Verification items for the finished model (mm, model axes). A direction names the side the tool comes from. Round coordinates to 2 decimals unless told otherwise and drop trailing zeros. Write each loop counter-clockwise with the first axis right and the second up, starting at its lowest first coordinate (ties: lowest second). Pieces come first, ordered by that corner, then holes. Notation, with made-up numbers: (59, -19.5) -> (91, -19.5) arc R14 cw to (91, -5.5) -> close; hole circle Ø11 at (-21.5, 2.25). An arc over 180 degrees is marked (long way). Use CSV: the item, a comma, the result in double quotes.
Autodesk Inventor part; units mm, degrees
ref_plane "Work Plane1" through (0, 0, 10) normal (0, 0, 1) x (1, 0, 0)
ref_plane "Work Plane3" through (3.9701, 45.8299, 26) normal (1, 0, 0) x (0, -1, 0)
ref_plane "Work Plane4" through (-34.8055, 8.3289, 16.6138) normal (0.7071068, -0.7071068, 0) x (0.7071068, 0.7071068, 0)
ref_plane "Work Plane1" through (0, 0, 10) normal (0, 0, 1) x (1, 0, 0)
sketch "Sketch1" plane through (0, 0, 10) normal (0, 0, 1) x (1, 0, 0)
  line L0 (-4.0299, -0.3538) -> (-2.2322, 1.4439) construction
  arc A0 (-1.4439, 2.2322) -> (-2.2322, 1.4439) centre (-0.9299, 0.9299) ccw construction
  line L1 (-1.4439, 2.2322) -> (0.3538, 4.0299) construction
  line L2 (-37.8299, 42.8299) -> (-37.8299, 37.8299) construction
  line L3 (-37.8299, 37.8299) -> (-42.9208, 37.8299) construction
  line L4 (-37.8299, 42.2137) -> (-37.8299, 45.8299) construction
  line L5 (-37.8299, 45.8299) -> (-4.0299, 45.8299) construction
  line L6 (-4.0299, 45.8299) -> (-4.0299, 42.2137) construction
  line L7 (-4.0299, 4.0299) -> (0.3538, 4.0299)
  circle A1 centre (-20.9299, 20.9299) radius 17.5
  line L8 (-20.9299, 58.9723) -> (17.1124, 20.9299) construction
  line L9 (17.1124, 20.9299) -> (-20.9299, -17.1124) construction
  line L10 (-20.9299, -17.1124) -> (-58.9723, 20.9299) construction
  line L11 (-58.9723, 20.9299) -> (-20.9299, 58.9723) construction
  line L12 (-20.9299, 58.9723) -> (-20.9299, -17.1124) construction
  line L13 (17.1124, 20.9299) -> (-58.9723, 20.9299) construction
  line L14 (-20.9299, 58.9723) -> (32.8701, 58.9723) construction
  line L15 (-43.4299, 43.4299) -> (1.5701, 43.4299) construction
  line L16 (1.5701, 43.4299) -> (1.5701, -1.5701) construction
  line L17 (1.5701, -1.5701) -> (-43.4299, -1.5701) construction
  line L18 (-43.4299, -1.5701) -> (-43.4299, 43.4299) construction
  line L19 (-43.4299, 43.4299) -> (1.5701, -1.5701) construction
  line L20 (1.5701, 43.4299) -> (-43.4299, -1.5701) construction
  line L21 (-43.4299, 5.3876) -> (-43.4299, 36.4723)
  line L22 (-43.4299, 36.4723) -> (-36.4723, 43.4299)
  line L23 (-36.4723, 43.4299) -> (-5.3876, 43.4299)
  line L24 (-5.3876, 43.4299) -> (1.5701, 36.4723)
  line L25 (1.5701, 36.4723) -> (1.5701, 5.3876)
  line L26 (1.5701, 5.3876) -> (-5.3876, -1.5701)
  line L27 (-5.3876, -1.5701) -> (-36.4723, -1.5701)
  line L28 (-36.4723, -1.5701) -> (-43.4299, 5.3876)
  line L29 (-4.0299, 42.2137) -> (-37.8299, 42.2137)
  line L30 (-4.0299, -0.3538) -> (-4.0299, 4.0299)
  circle A2 centre (-20.9299, 20.9299) radius 1.4
  line L31 (-10.9299, 10.9299) -> (-30.9299, 10.9299) construction
  line L32 (-30.9299, 10.9299) -> (-30.9299, 30.9299) construction
  line L33 (-30.9299, 30.9299) -> (-10.9299, 30.9299) construction
  line L34 (-10.9299, 30.9299) -> (-10.9299, 10.9299) construction
  line L35 (-10.9299, 10.9299) -> (-30.9299, 30.9299) construction
  line L36 (-30.9299, 10.9299) -> (-10.9299, 30.9299) construction
  circle A3 centre (-30.9299, 30.9299) radius 1.4
  circle A4 centre (-30.9299, 10.9299) radius 1.4
  circle A5 centre (-10.9299, 10.9299) radius 1.4
  line L37 (-45.8299, 37.8299) -> (-42.0723, 37.8299) construction
  line L38 (-42.1723, 37.7299) -> (-45.8299, 37.7299)
  line L39 (-45.8299, 37.7299) -> (-45.8299, 4.1299)
  line L40 (-45.8299, 4.1299) -> (-42.1723, 4.1299)
  line L41 (-42.1723, 4.1299) -> (-42.1723, 37.7299)
  line L42 (-45.8299, 4.0299) -> (-42.0723, 4.0299) construction
  line L43 (-45.8299, 37.8299) -> (-42.0723, 37.8299)
  line L44 (-37.7299, 45.8299) -> (-4.1299, 45.8299)
  line L45 (-4.1299, 45.8299) -> (-4.1299, 42.1723)
  line L46 (-4.1299, 42.1723) -> (-37.7299, 42.1723)
  line L47 (-37.7299, 42.1723) -> (-37.7299, 45.8299)
  line L48 (0.4701, 37.8299) -> (0.4701, 4.0299) construction
  line L49 (0.4701, 4.0299) -> (3.9701, 4.0299) construction
  line L50 (3.9701, 37.8299) -> (3.9701, 4.0299) construction
  line L51 (0.4701, 37.8299) -> (3.9701, 37.8299) construction
  line L52 (-45.8299, -3.9701) -> (-4.0299, -3.9701) construction
  line L53 (0.3124, 37.7299) -> (3.9701, 37.7299)
  line L54 (3.9701, 37.7299) -> (3.9701, 4.1299)
  line L55 (3.9701, 4.1299) -> (0.3124, 4.1299)
  line L56 (0.3124, 4.1299) -> (0.3124, 37.7299)
  line L57 (-4.1713, -0.3538) -> (-37.7299, -0.3538)
  line L58 (-37.7299, -0.3538) -> (-37.7299, -3.9701)
  line L59 (-37.7299, -3.9701) -> (-4.1713, -3.9701)
  line L60 (-4.1713, -3.9701) -> (-4.1713, -0.3538)
  point P0 (-37.8299, 4.0299)
  dimension "d18" = 53.8
  dimension "d19" = 45
  dimension "d20" = 53.8
  dimension "d21" = 45
  dimension "d22" = 45
  dimension "d30" = 20
  dimension "d31" = 20
  dimension "d32" = 2.8
  dimension "d33" = 2.8
  dimension "d34" = 2.8
  dimension "d35" = 2.8
  dimension "d36" = 0.1
  dimension "d37" = 0.1
  dimension "d38" = 0.1
  dimension "d39" = 0.1
extrude "Extrusion1" add sketch "Sketch1" along normal blind 5 contours L30 L26 L57 L28 L41 L22 L46 L24 L56 L7 | L7 L26 L30 | L56 L24 L25 L26 | L26 L25 L24 L53 L54 L55 | L60 L59 L58 L57 L28 L27 L26 | L26 L27 L28 L57 | L46 L22 L29 L24 | L24 L29 L45 | L40 L39 L38 L22 L21 L28 | L28 L21 L22 L41 | L29 L22 L23 L24 | L24 L23 L22 L29 L47 L44 L45 | L47 L29 L22 | A1 | A2 | A3 | A4 | A5
sketch "Sketch4" plane through (0, 0, 15) normal (0, 0, 1) x (1, 0, 0)
  line L0 (-37.7299, 42.1723) -> (-42.1723, 37.7299)
  line L1 (-42.1723, 37.7299) -> (-45.8299, 37.7299)
  line L2 (-45.8299, 37.7299) -> (-45.8299, 4.1299)
  line L3 (-45.8299, 4.1299) -> (-42.1723, 4.1299)
  line L4 (-42.1723, 4.1299) -> (-37.6885, -0.3538)
  line L5 (-37.6885, -0.3538) -> (-37.7299, -0.3538)
  line L6 (-37.7299, -0.3538) -> (-37.7299, -3.9701)
  line L7 (-37.7299, -3.9701) -> (-4.1713, -3.9701)
  line L8 (-4.1713, -3.9701) -> (-4.1713, -0.3538)
  line L9 (-4.1713, -0.3538) -> (0.3124, 4.1299)
  line L10 (0.3124, 4.1299) -> (3.9701, 4.1299)
  line L11 (3.9701, 4.1299) -> (3.9701, 37.7299)
  line L12 (3.9701, 37.7299) -> (0.3124, 37.7299)
  line L13 (0.3124, 37.7299) -> (-4.1299, 42.1723)
  line L14 (-4.1299, 42.1723) -> (-4.1299, 45.8299)
  line L15 (-4.1299, 45.8299) -> (-37.7299, 45.8299)
  line L16 (-37.7299, 45.8299) -> (-37.7299, 42.1723)
  line L17 (-45.8299, 37.7299) -> (-45.8299, 4.1299)
  line L18 (-45.8299, 7.911) -> (-7.911, 45.8299)
  line L19 (-45.8299, 7.911) -> (7.7955, 7.911) construction
  line L20 (-7.911, 45.8299) -> (-14.9821, 45.8299)
  line L21 (-4.1299, 45.8299) -> (-37.7299, 45.8299)
  line L22 (-14.9821, 45.8299) -> (-45.8299, 14.9821)
  line L23 (-45.8299, 7.911) -> (-45.8299, 14.9821)
  circle A0 centre (-40.9299, 0.9299) radius 1.1933
  line L24 (0.3124, 37.7299) -> (-4.1299, 42.1723)
  point P0 (0, 0)
  dimension "d40" = 45
  dimension "d41" = 5
extrude "Extrusion4" add sketch "Sketch4" along normal blind 27.5 contours L15 L18 L2 L22
sketch "Sketch5" plane through (-45.8299, 14.9821, 15) normal (-0.7071068, 0.7071068, 0) x (-0.7071068, -0.7071068, 0)
  line L0 (0, 0) -> (-43.6254, 0)
  line L1 (0, 0) -> (0, 27.5)
  line L2 (-43.6254, 27.5) -> (0, 27.5)
  line L3 (-43.6254, 0) -> (-43.6254, 27.5)
  circle A0 centre (-21.8127, 5.6873) radius 21.8127
  line L4 (-6.8127, 24) -> (-36.8127, 24) construction
  line L5 (-36.8127, 24) -> (-36.8127, 4) construction
  line L6 (-36.8127, 4) -> (-6.8127, 4) construction
  line L7 (-6.8127, 4) -> (-6.8127, 24) construction
  line L8 (-6.8127, 24) -> (-36.8127, 4) construction
  line L9 (-36.8127, 24) -> (-6.8127, 4) construction
  point P0 (-21.8127, -15)
  point P1 (-21.8127, 14)
  dimension "d44" = 30
  dimension "d45" = 20
hole "Hole1" at (-19.7994, 41.0126, 39) at (-19.7994, 41.0126, 19) at (-41.0126, 19.7994, 39) at (-30.406, 30.406, 29) direction (0.7071068, -0.7071068, 0) diameter 2.8 depth 12
sketch "Sketch6" plane through (-37.7299, -3.9701, 10) normal (0, -1, 0) x (1, 0, 0)
  circle A0 centre (-3.2, 36.9) radius 1.45
  circle A1 centre (36.8, 36.9) radius 1.45
  line L0 (-6.1, 0) -> (-6.1, 39.8)
  line L1 (-0.1, 0) -> (-6.1, 0)
  line L2 (-0.1, 33.8) -> (-0.1, 0)
  line L3 (33.7, 33.8) -> (-0.1, 33.8)
  line L4 (33.7, 33.8) -> (33.7, 0)
  line L5 (39.7, 0) -> (33.7, 0)
  line L6 (39.7, 39.8) -> (39.7, 0)
  line L7 (-6.1, 39.8) -> (39.7, 39.8)
  circle A2 centre (16.8, 16.9) radius 16.9
  circle A3 centre (16.8, 16.9) radius 14.9
  line L8 (-0.1, 16.9) -> (-0.1, 0)
  line L9 (0, 0) -> (33.5586, 0)
  line L10 (0.0414, 0) -> (-4.4423, 0)
  line L11 (33.5586, 0) -> (0.0414, 0)
  line L12 (33.7, 16.9) -> (33.5586, 0)
  point P0 (37.7299, -10)
  dimension "d53" = 2
extrude "Extrusion5" cut sketch "Sketch6" against normal up to surface contours A3 surface through (-45.8299, 7.911, 15) normal (0.7071068, -0.7071068, 0)
ref_plane "Work Plane3" through (3.9701, 45.8299, 26) normal (1, 0, 0) x (0, -1, 0)
sketch "Sketch7" plane through (3.9701, 45.8299, 26) normal (1, 0, 0) x (0, -1, 0)
  line L0 (41.8, -17.8) -> (41.8, 16)
  line L1 (8, -17.8) -> (41.8, -17.8)
  line L2 (8, -17.8) -> (8, 16)
  circle A0 centre (24.9, -0.9) radius 16.9
  circle A1 centre (24.9, -0.9) radius 14.9
  point P0 (45.8299, 26)
  dimension "d56" = 2
ref_plane "Work Plane4" through (-34.8055, 8.3289, 16.6138) normal (0.7071068, -0.7071068, 0) x (0.7071068, 0.7071068, 0)
extrude "Extrusion6" cut sketch "Sketch7" against normal up to surface contours A1 surface through (-45.8299, 7.911, 15) normal (0.7071068, -0.7071068, 0)
sketch "Skizze8" plane through (0, 0, 10) normal (0, 0, -1) x (-1, 0, 0)
  line L0 (42.1723, 37.7299) -> (37.7299, 42.1723)
  line L1 (37.7299, 45.8299) -> (37.7299, 42.1723)
  line L2 (4.1299, 45.8299) -> (37.7299, 45.8299) construction
  line L3 (4.1299, 42.1723) -> (4.1299, 45.8299)
  line L4 (4.1299, 42.1723) -> (-0.3124, 37.7299)
  line L5 (-3.9701, 37.7299) -> (-0.3124, 37.7299)
  line L6 (-3.9701, 4.1299) -> (-3.9701, 37.7299) construction
  line L7 (-0.3124, 4.1299) -> (-3.9701, 4.1299)
  line L8 (-0.3124, 4.1299) -> (4.1713, -0.3538)
  line L9 (4.1713, -3.9701) -> (4.1713, -0.3538)
  line L10 (37.7299, -3.9701) -> (4.1713, -3.9701) construction
  line L11 (37.7299, -0.3538) -> (37.7299, -3.9701)
  line L12 (37.6885, -0.3538) -> (37.7299, -0.3538)
  line L13 (37.6885, -0.3538) -> (42.1723, 4.1299)
  line L14 (45.8299, 4.1299) -> (42.1723, 4.1299)
  line L15 (45.8299, 37.7299) -> (45.8299, 4.1299) construction
  line L16 (42.1723, 37.7299) -> (45.8299, 37.7299)
  line L17 (46.0299, 3.9299) -> (42.2551, 3.9299)
  line L18 (42.2551, 3.9299) -> (37.9299, -0.3953)
  line L19 (37.9299, -0.3953) -> (37.9299, -4.1701)
  line L20 (37.9299, -4.1701) -> (3.9713, -4.1701) construction
  line L21 (3.9713, -4.1701) -> (3.9713, -0.4367)
  line L22 (3.9713, -0.4367) -> (-0.3953, 3.9299)
  line L23 (-0.3953, 3.9299) -> (-4.1701, 3.9299)
  line L24 (-4.1701, 3.9299) -> (-4.1701, 37.9299) construction
  line L25 (-4.1701, 37.9299) -> (-0.3953, 37.9299)
  line L26 (-0.3953, 37.9299) -> (3.9299, 42.2551)
  line L27 (3.9299, 42.2551) -> (3.9299, 46.0299)
  line L28 (3.9299, 46.0299) -> (37.9299, 46.0299) construction
  line L29 (37.9299, 46.0299) -> (37.9299, 42.2551)
  line L30 (37.9299, 42.2551) -> (42.2551, 37.9299)
  line L31 (42.2551, 37.9299) -> (46.0299, 37.9299)
  line L32 (46.0299, 37.9299) -> (46.0299, 3.9299) construction
  line L33 (37.7299, 45.8299) -> (37.7299, 42.1723)
  line L34 (37.7299, 45.8299) -> (37.9299, 45.8299)
  line L35 (42.1723, 37.7299) -> (45.8299, 37.7299)
  line L36 (45.8299, 37.7299) -> (45.8299, 37.9299)
  line L37 (45.8299, 4.1299) -> (45.8299, 3.9299)
  line L38 (37.7299, -3.9701) -> (4.1713, -3.9701)
  line L39 (37.7299, -3.9701) -> (37.9299, -3.9701)
  line L40 (4.1713, -3.9701) -> (3.9713, -3.9701)
  line L41 (-3.9701, 4.1299) -> (-3.9701, 3.9299)
  line L42 (-3.9701, 37.7299) -> (-0.3124, 37.7299)
  line L43 (-3.9701, 37.7299) -> (-3.9701, 37.9299)
  line L44 (4.1299, 42.1723) -> (4.1299, 45.8299)
  line L45 (4.1299, 45.8299) -> (3.9299, 45.8299)
  point P0 (0, 0)
  dimension "d59" = 0.2
extrude "IM_offset" add sketch "Skizze8" against normal up to surface (5 mm away)
properties part number "20_Cube_Insert_Kinematic_Mirrormount_45_base_v3_aaa"
Q1. Mould release check, pull along Y, two halves, no side actions. Record for faces 4 (the flat face through (-21, -3.97, 11)), 5 (the flat face through (-37.93, -2, 12)), 6 (the cylindrical face through (-6, 21, 12)): released by +Y, released by -Y, zero draft, split by the parting line, or undercut.
Filled in:
face 4,"released by -Y"
face 5,"zero draft"
face 6,"undercut"
Q2. Section check D-D (y = 22.5). Record the cut outline in (x, z), plus the area to 3 significant figures.
Filled in:
outline,"(-45.83, 10) -> (3.97, 10) -> (3.97, 12.08) -> (-19.36, 12.08) arc R14.9 cw to (-22.5, 12.08) -> (-31.24, 12.08) -> (-31.24, 42.5) -> (-38.31, 42.5) -> (-38.31, 15) -> (-45.83, 15) -> close"
area,"341 mm²"
Q3. Go/stop test with flat-tipped pins: P1, Ø4, axis at x = 2, z = 13.5, coming from the -Y side; P2, Ø2, axis at x = -37.5, z = 28, coming from the +Y side; P3, Ø10, axis at y = 35.5, z = 35.5, coming from the -X side. Record where each tip stops, or that it passes through.
Filled in:
P1,"y = 3.53"
P2,"y = 24.31"
P3,"x = -30.31"
Q4. Section check B-B (x = -34). Record the cut outline in (y, z).
Filled in:
outline,"(-3.97, 10) -> (45.83, 10) -> (45.83, 15) -> (26.81, 15) -> (26.81, 42.5) -> (19.74, 42.5) -> (19.74, 12.05) arc R14.9 cw to (11.96, 15) -> (-3.97, 15) -> close"
Q5. Section check C-C (y = 14). Record the cut outline in (x, z).
Filled in:
outline,"(-45.83, 10) -> (3.97, 10) -> (3.97, 13.71) -> (-14, 13.71) arc R14.9 cw to (-27.86, 13.71) -> (-39.74, 13.71) -> (-39.74, 42.5) -> (-45.83, 42.5) -> close"
Q6. Access from +Z, -Z, +X, -X, +Y, -Y to the whole of each face (thin tool, end or side, straight path). Record for faces 1 (the flat face through (-3.971, -2, 12)), 2 (the flat face through (-6, 6, 15)), 3 (the flat face through (-34, 34, 15)).
Filled in:
face 1,"+Z, -Z, +X, -Y"
face 2,"+Z, +X, -Y"
face 3,"+Z, -X, +Y"
Q7. Material ranges on L1, parallel to Z at x = -30, y = 38.5; L2, parallel to Y at x = -29, z = 29.5; L3, parallel to X at y = 12.5, z = 14.5, recorded low to high.
Filled in:
L1,"10 to 15"
L2,"24.74 to 27.15, 30.85 to 31.81"
L3,"-45.83 to -29.19, -12.67 to 3.97"
Q8. Section check A-A (z = 14). Record the cut outline in (x, y).
Filled in:
outline,"(-45.83, 3.93) -> (-42.26, 3.93) -> (-37.93, -0.4) -> (-37.93, -3.97) -> (-28.39, -3.97) -> (-28.39, 13.47) -> (-40.27, 13.47) -> (-13.47, 40.27) -> (-13.47, 28.39) -> (3.97, 28.39) -> (3.97, 37.93) -> (0.4, 37.93) -> (-3.93, 42.26) -> (-3.93, 45.83) -> (-37.93, 45.83) -> (-37.93, 42.26) -> (-42.26, 37.93) -> (-45.83, 37.93) -> close; (-13.47, -3.97) -> (-3.97, -3.97) -> (-3.97, -0.44) -> (0.4, 3.93) -> (3.97, 3.93) -> (3.97, 13.47) -> (-13.47, 13.47) -> close"
